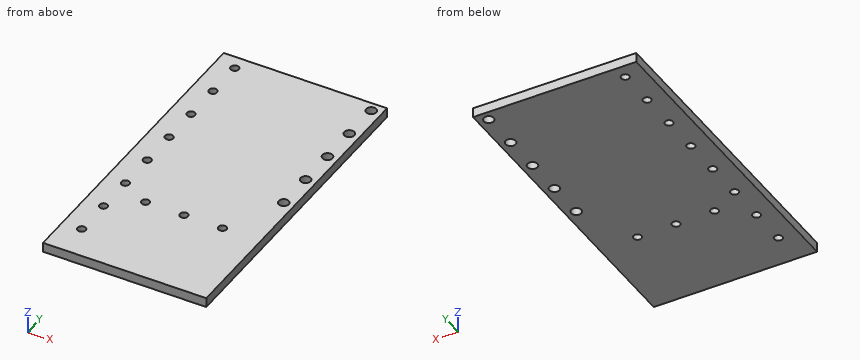
Autodesk Inventor part; units mm, degrees
ref_plane "YZ Plane" through (0, 0, 0) normal (1, 0, 0) x (0, 1, 0)
ref_plane "XZ Plane" through (0, 0, 0) normal (0, 1, 0) x (-1, 0, 0)
ref_plane "XY Plane" through (0, 0, 0) normal (0, 0, 1) x (1, 0, 0)
ref_plane "Work Plane3" through (0, 0, 0) normal (0, 0, 1) x (1, 0, 0)
sketch "Sketch1" plane through (0, 0, 0) normal (0, 0, 1) x (1, 0, 0)
  line L0 (-755.65, -71.0123) -> (-755.65, -75.0128)
  line L1 (-57.15, -75.0128) -> (-755.65, -75.0128)
  line L2 (-57.15, -75.0128) -> (-57.15, -71.0123)
  line L3 (-57.15, -71.0123) -> (-755.65, -71.0123)
  line L4 (-57.15, -78.9498) -> (-755.65, -78.9498)
  line L5 (-755.65, -78.9498) -> (-647.9579, -78.9498)
  line L6 (-647.9579, -78.9498) -> (-647.9579, 130.9029)
  line L7 (-647.9579, 130.9029) -> (-755.65, 130.9029)
  line L8 (-755.65, 130.9029) -> (-755.65, -78.9498)
  point P0 (0, 0)
extrude "Extrusion1" add sketch "Sketch1" along normal blind 6.35 contours L3 L6 L1 L0 | L8 L7 L6 L3 | L1 L6 L4 L8
sketch "Sketch3" plane through (0, 0, 6.35) normal (0, 0, 1) x (1, 0, 0)
  point P0 (0, 0)
sketch "Sketch4" plane through (0, 0, 6.35) normal (0, 0, 1) x (1, 0, 0)
  circle A0 centre (-654.685, 22.86) radius 3.3528
  circle A1 centre (-654.685, 48.26) radius 3.3528
  circle A2 centre (-654.685, 73.66) radius 3.3528
  circle A3 centre (-654.685, 99.06) radius 3.3528
  circle A4 centre (-654.685, 124.46) radius 3.3528
  line L0 (-663.448, 15.875) -> (-648.335, 15.875) construction
  line L1 (-648.335, 133.985) -> (-648.335, 15.875) construction
  line L2 (-648.335, 133.985) -> (-651.51, 137.16) construction
  line L3 (-663.448, 137.16) -> (-651.51, 137.16) construction
  line L4 (-663.448, 137.16) -> (-663.448, 15.875) construction
  line L5 (-663.448, 137.16) -> (-663.448, 15.875)
  point P0 (0, 0)
extrude "Extrusion2" cut sketch "Sketch4" against normal blind 6.35
sketch "Sketch5" plane through (0, 0, 6.35) normal (0, 0, 1) x (1, 0, 0)
  line L0 (-736.6, -3.937) -> (-736.6, -22.225)
  line L1 (-460.375, -22.225) -> (-736.6, -22.225)
  line L2 (-460.375, -22.225) -> (-457.2, -19.05)
  line L3 (-457.2, -3.937) -> (-457.2, -19.05)
  line L4 (-736.6, -3.937) -> (-457.2, -3.937)
  circle A0 centre (-469.9, -15.875) radius 2.667
  circle A1 centre (-495.3, -15.875) radius 2.667
  circle A2 centre (-520.7, -15.875) radius 2.667
  circle A3 centre (-546.1, -15.875) radius 2.667
  circle A4 centre (-571.5, -15.875) radius 2.667
  circle A5 centre (-596.9, -15.875) radius 2.667
  circle A6 centre (-622.3, -15.875) radius 2.667
  circle A7 centre (-647.7, -15.875) radius 2.667
  circle A8 centre (-673.1, -15.875) radius 2.667
  circle A9 centre (-698.5, -15.875) radius 2.667
  circle A10 centre (-723.9, -15.875) radius 2.667
  circle A11 centre (-742.95, 476.947) radius 2.667
  circle A12 centre (-742.95, 451.547) radius 2.667
  circle A13 centre (-742.95, 426.147) radius 2.667
  circle A14 centre (-742.95, 400.747) radius 2.667
  circle A15 centre (-742.95, 375.347) radius 2.667
  circle A16 centre (-742.95, 349.947) radius 2.667
  circle A17 centre (-742.95, 324.547) radius 2.667
  circle A18 centre (-742.95, 299.147) radius 2.667
  circle A19 centre (-742.95, 273.747) radius 2.667
  circle A20 centre (-742.95, 248.347) radius 2.667
  circle A21 centre (-742.95, 222.947) radius 2.667
  circle A22 centre (-742.95, 197.547) radius 2.667
  circle A23 centre (-742.95, 172.147) radius 2.667
  circle A24 centre (-742.95, 146.747) radius 2.667
  circle A25 centre (-742.95, 121.347) radius 2.667
  circle A26 centre (-742.95, 95.947) radius 2.667
  circle A27 centre (-742.95, 70.547) radius 2.667
  circle A28 centre (-742.95, 45.147) radius 2.667
  circle A29 centre (-742.95, 19.747) radius 2.667
  circle A30 centre (-742.95, -5.653) radius 2.667
  circle A31 centre (-742.95, -31.053) radius 2.667
  circle A32 centre (-742.95, -56.453) radius 2.667
  line L5 (-736.6, 496.0909) -> (-751.713, 496.0909)
  line L6 (-751.713, -75.5081) -> (-751.713, 496.0909)
  line L7 (-751.713, -75.5081) -> (-736.6, -75.5081)
  line L8 (-736.6, 496.0909) -> (-736.6, -75.5081)
  point P0 (0, 0)
extrude "Extrusion3" cut sketch "Sketch5" against normal blind 6.35 contours A8 | A9 | A10 | A25 | A26 | A27 | A28 | A29 | A30 | A31 | A32
properties part number "Aluminum Mounting Plate"
Geometry: final body of the model. Coordinates: model frame, mm. Round coordinates to 2 decimals unless told otherwise and drop trailing zeros. Order: outer loops, then holes, each group sorted by start corner. A loop starts at its lowest first (then second) coordinate and runs counter-clockwise, first axis right, second up. Notation, with made-up numbers: (33, -7) -> (42, -7) arc R21 cw to (42, 3) -> close; hole circle Ø5 at (-30.5, 59.25). An arc over 180 degrees is marked (long way). Put each result on its own line as item: value. Start each with the question number.
Q1. First-contact query: pin 1 (5 mm diameter, centred on x = -723.9, y = -15.875, fed in from -Z). Flat tip, straight axial feed; report the tip coordinate or a pass-through.
Q2. Section A-A on x = -673.1. Return the cut outline in (y, z), and give its area (3 significant figures).
Q3. Line query: probe 1 along Y at (x, z) = (-655, 1.75); probe 2 along X at (y, z) = (20.5, 4); probe 3 along Y at (x, z) = (-698.5, 3.25). Output: solid intervals per line, ascending.
Q4. Section B-B on z = 2. Give the number of separate pieces and of enclosed holes in the cut face, and give its area (3 significant figures).
Ans:
1. pin 1: passes through
2. outline: (-78.95, 0) -> (-18.54, 0) -> (-18.54, 6.35) -> (-78.95, 6.35) -> close; (-13.21, 0) -> (130.9, 0) -> (130.9, 6.35) -> (-13.21, 6.35) -> close
2. area: 1,300 mm2
3. probe 1: y = -78.95 to 19.52, 26.2 to 44.92, 51.6 to 70.32, 77 to 95.72, 102.4 to 121.12, 127.8 to 130.9
3. probe 2: x = -755.65 to -745.51, -740.39 to -657.07, -652.3 to -647.96
3. probe 3: y = -78.95 to -18.54, -13.21 to 130.9
4. separate pieces: 1
4. enclosed holes: 16
4. area: 22,200 mm2
